```python
from build123d import *

# Parameters (mm, degrees)
SKETCH1_W            = 178
SKETCH1_H            = 150
BOSS_EXTRUDE1_DEPTH  = 6
SKETCH2_W            = 6
SKETCH2_H            = 25
CUT_EXTRUDE1_DEPTH   = 6
LPATTERN1_COUNT      = 3
LPATTERN1_PITCH      = 50
LPATTERN1_COUNT_DIR2 = 2
LPATTERN1_PITCH_DIR2 = 172
SKETCH3_W            = 15
SKETCH3_H            = 6
CUT_EXTRUDE2_DEPTH   = 233.851884253


with BuildPart() as part:
    # Sketch1 → Boss-Extrude1 (new body)
    with BuildSketch(Plane.XY):
        with Locations((-89, 75)):
            Rectangle(SKETCH1_W, SKETCH1_H)
    extrude(amount=BOSS_EXTRUDE1_DEPTH)

    # Sketch2 → Cut-Extrude1 (cut)
    with BuildSketch(Plane.XY.offset(6)):
        with Locations((-175, 112.5)):
            Rectangle(SKETCH2_W, SKETCH2_H)
    cut_extrude1 = extrude(amount=-CUT_EXTRUDE1_DEPTH, mode=Mode.SUBTRACT)

    # LPattern1: Cut-Extrude1 3 × 2
    with Locations(*[(j * LPATTERN1_PITCH_DIR2, -i * LPATTERN1_PITCH, 0) for i in range(LPATTERN1_COUNT) for j in range(LPATTERN1_COUNT_DIR2) if (i, j) != (0, 0)]):
        add(cut_extrude1, mode=Mode.SUBTRACT)

    # Sketch3 → Cut-Extrude2 (cut, through all)
    with BuildSketch(Plane.XY.offset(6)):
        with Locations((-23.5, 3)):
            Rectangle(SKETCH3_W, SKETCH3_H)
        with Locations((-154.5, 3)):
            Rectangle(SKETCH3_W, SKETCH3_H)
    extrude(amount=-CUT_EXTRUDE2_DEPTH, mode=Mode.SUBTRACT)


solid = part.part
```
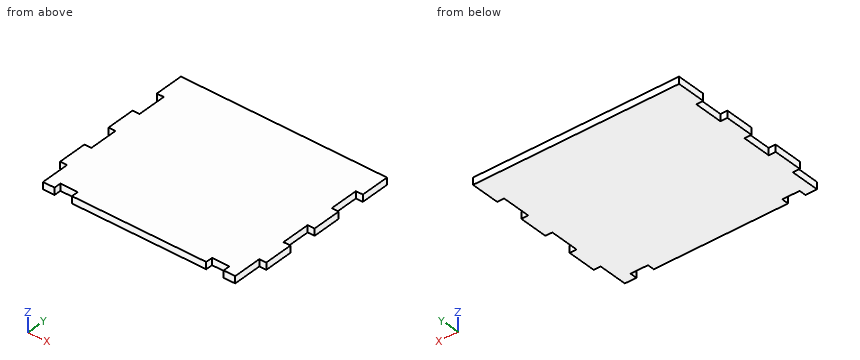
Check sheet for the modelled part. Datum: model origin and axes. Units: mm. Round coordinates to 2 decimals unless told otherwise and drop trailing zeros. Order: outer loops, then holes, each group sorted by start corner. A loop starts at its lowest first (then second) coordinate and runs counter-clockwise, first axis right, second up.
1) Section check B-B (x = -150.5). Record the boundary of the cut face in (y, z).
2) Go/stop test with flat-tipped pins: pin 1 Ø3 at (y, z) = (12.5, 3) entering from -X; pin 2 Ø1.8 at (y, z) = (4, 2) entering from +X; pin 3 Ø1.8 at (x, z) = (-176, 2) entering from -Y. Record where each tip stops, or that it passes through.
3) Section check C-C (y = 60.5). Record the boundary of the cut face in (x, z), and give its area (3 significant figures).
4) Scan lines: line 1 (X direction, y = 63, z = 5.05); line 2 (Y direction, x = -20, z = 2.3). Record each from-to range of solid material in increasing order.
Result:
1. outline: (6, 0) - (150, 0) - (150, 6) - (6, 6) - close
2. pin 1: stops at x = -172
2. pin 2: stops at x = -6
2. pin 3: stops at y = 25
3. outline: (-172, 0) - (-6, 0) - (-6, 6) - (-172, 6) - close
3. area: 996 mm2
4. line 1: x = -172 to -6
4. line 2: y = 6 to 150
